Work out the finished part from the listing and answer in its coordinate system (mm). A direction names the side the tool comes from. Give positions to 0.01 mm unless a question says otherwise; leave off trailing zeros. Write each loop counter-clockwise with the first axis right and the second up, starting at its lowest first coordinate (ties: lowest second). Pieces come first, ordered by that corner, then holes. Notation, with made-up numbers: (11, 39.25) -> (55, 39.25) arc R21 ccw to (55, 45.25) -> close; hole circle Ø10 at (57.25, 27). An arc over 180 degrees is marked (long way). Use a Markdown table: item, result. Add a question column.
Q1. Section B-B, the plane x = -9.5 is taken. Give the vertices of the cut face in (y, z).
Q2. Consider line 1 (X direction, y = 42, z = -20); line 2 (X direction, y = -46, z = 20); line 3 (X direction, y = -21, z = 30). Determine where each line is inside the solid, lowest interval first.
Q3. Section D-D, the plane z = -25 is taken. Give the vertices of the cut face in (x, y).
Q4. This flat-tipped pin is pushed along its axis until it touches: pin 1 Ø9.5 at (y, z) = (25, 25) entering from +X. Where does it stop, or does it pass through?
Q5. Section C-C, the plane x = -25 is taken. Give the vertices of the cut face in (y, z).
Q6. Section A-A, the plane z = -37 is taken. Give the vertices of the cut face in (x, y), plus the area to 3 significant figures.
Q7. For a pull along Z with two mould halves and no side action, classify faces 1 (the face through (18.2, -44.9, 17.6)), 2 (the face through (-1, 40, -1)), 3 (the face through (20.904, 25.18, 46.302)) as pulls with the +Z half, pulls with the -Z half, needs draft (parallel to the pull), parting line crosses it, or undercut.
Q8. For faces 4 (the face through (-42.5, 1, 1)), 5 (the face through (18.2, 45.1, 17.6)), determine the directions among +Z, -Z, +X, -X, +Y, -Y from which every point of the face is accessible in a straight line to the end or side of a thin tool.
from build123d import *

# Parameters (mm, degrees)
SKETCH1_W           = 100
SKETCH1_H           = 100
BOSS_EXTRUDE1_DEPTH = 50
SKETCH2_R           = 4.1
CUT_EXTRUDE1_DEPTH  = 123.474487139
SKETCH3_R           = 4.1
CUT_EXTRUDE2_DEPTH  = 123.474487139
SKETCH4_R           = 3
SKETCH4_R_2         = 3.25
CUT_EXTRUDE3_DEPTH  = 123.474487139
SKETCH8_W           = 85
SKETCH8_H           = 85
CUT_EXTRUDE4_DEPTH  = 40


with BuildPart() as part:
    # Sketch1 → Boss-Extrude1 (new, symmetric)
    with BuildSketch(Plane.XY):
        Rectangle(SKETCH1_W, SKETCH1_H)
    extrude(amount=BOSS_EXTRUDE1_DEPTH, both=True)

    # Sketch2 → Cut-Extrude1 (cut, through all)
    with BuildSketch(Plane.XY.offset(50)):
        with Locations((-25, 25)):
            Circle(SKETCH2_R)
        with Locations((25, 25)):
            Circle(SKETCH2_R)
        with Locations((25, -25)):
            Circle(SKETCH2_R)
        with Locations((-25, -25)):
            Circle(SKETCH2_R)
    extrude(amount=-CUT_EXTRUDE1_DEPTH, mode=Mode.SUBTRACT)

    # Sketch3 → Cut-Extrude2 (cut, through all)
    with BuildSketch(Plane(origin=(50, 0, 0), x_dir=(0, 0, -1), z_dir=(1, 0, 0))):
        with Locations((-25, 25)):
            Circle(SKETCH3_R)
        with Locations((25, 25)):
            Circle(SKETCH3_R)
        with Locations(Location((25, -25, 0), (0, 0, 90))):
            Circle(SKETCH3_R)
        with Locations(Location((-25, -25, 0), (0, 0, 270))):
            Circle(SKETCH3_R)
    extrude(amount=-CUT_EXTRUDE2_DEPTH, mode=Mode.SUBTRACT)

    # Sketch4 → Cut-Extrude3 (cut, through all)
    with BuildSketch(Plane(origin=(0, 50, 0), x_dir=(1, 0, 0), z_dir=(0, 1, 0))):
        with Locations(Location((-20, 20, 0), (0, 0, 270))):
            Circle(SKETCH4_R)
        with Locations(Location((20, -20, 0), (0, 0, 270))):
            Circle(SKETCH4_R)
        with Locations(Location((20, 20, 0), (0, 0, 270))):
            Circle(SKETCH4_R_2)
        with Locations(Location((-20, -20, 0), (0, 0, 270))):
            Circle(SKETCH4_R_2)
    extrude(amount=-CUT_EXTRUDE3_DEPTH, mode=Mode.SUBTRACT)

    # Sketch8 → Cut-Extrude4 (cut, symmetric)
    with BuildSketch(Plane(origin=(0, 0, 0), x_dir=(1, 0, 0), z_dir=(0, 1, 0))):
        Rectangle(SKETCH8_W, SKETCH8_H)
    extrude(amount=CUT_EXTRUDE4_DEPTH, both=True, mode=Mode.SUBTRACT)


solid = part.part
Result set:
| question | item | result |
|---|---|---|
| 1 | outline | (-50, -50) -> (50, -50) -> (50, 50) -> (-50, 50) -> close; hole (-40, -42.5) -> (40, -42.5) -> (40, 42.5) -> (-40, 42.5) -> close |
| 2 | line 1 | x = -50 to -23, -17 to 16.75, 23.25 to 50 |
| 2 | line 2 | x = -50 to -23.25, -16.75 to 17, 23 to 50 |
| 2 | line 3 | x = -50 to -42.5, 42.5 to 50 |
| 3 | outline | (-50, -50) -> (50, -50) -> (50, -29.1) -> (42.5, -29.1) -> (42.5, -40) -> (-42.5, -40) -> (-42.5, -29.1) -> (-50, -29.1) -> close; (-50, -20.9) -> (-42.5, -20.9) -> (-42.5, 20.9) -> (-50, 20.9) -> close; (-50, 29.1) -> (-42.5, 29.1) -> (-42.5, 40) -> (42.5, 40) -> (42.5, 29.1) -> (50, 29.1) -> (50, 50) -> (-50, 50) -> close; (42.5, -20.9) -> (50, -20.9) -> (50, 20.9) -> (42.5, 20.9) -> close |
| 4 | pin 1 | stops at x = 50 |
| 5 | outline | (-50, -50) -> (-29.1, -50) -> (-29.1, -42.5) -> (-40, -42.5) -> (-40, 42.5) -> (-29.1, 42.5) -> (-29.1, 50) -> (-50, 50) -> close; (-20.9, -50) -> (20.9, -50) -> (20.9, -42.5) -> (-20.9, -42.5) -> close; (-20.9, 42.5) -> (20.9, 42.5) -> (20.9, 50) -> (-20.9, 50) -> close; (29.1, -50) -> (50, -50) -> (50, 50) -> (29.1, 50) -> (29.1, 42.5) -> (40, 42.5) -> (40, -42.5) -> (29.1, -42.5) -> close |
| 6 | outline | (-50, -50) -> (50, -50) -> (50, 50) -> (-50, 50) -> close; hole (-42.5, -40) -> (42.5, -40) -> (42.5, 40) -> (-42.5, 40) -> close |
| 6 | area | 3,200 mm2 |
| 7 | face 1 | undercut |
| 7 | face 2 | undercut |
| 7 | face 3 | needs draft |
| 8 | face 4 | none |
| 8 | face 5 | +Y, -Y |
